Geometry check sheet. Reference: drawing and pictorial views, mm from the part's lowest x, y, z. Round coordinates to 2 decimals unless told otherwise and drop trailing zeros. Write each loop counter-clockwise with the first axis right and the second up, starting at its lowest first coordinate (ties: lowest second). Pieces come first, ordered by that corner, then holes. Notation, with made-up numbers: M 5.25,21 L 56.25,21 A22 ccw 56.25,37 Z; hole C -22,66 d3. An arc over 180 degrees is marked long. One line per item, written item: value. Start each with the question number.
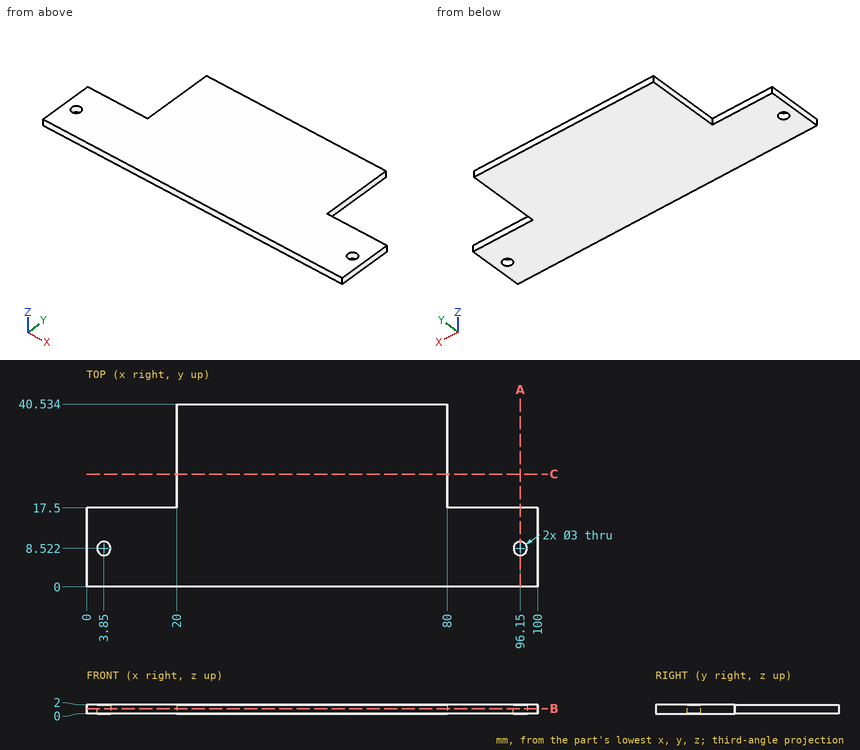
1) Gauge pin test, flat ends, axial feed: pin 1 Ø0.6 at (x, z) = (89, 1) entering from +Y; pin 2 Ø2.5 at (x, y) = (3.85, 8.52) entering from -Z. Record the tip position at first contact, or that the pin passes through.
2) Cross-section at A-A (x = 96.15). Record the boundary of the cut face in (y, z).
3) Cross-section at B-B (z = 1.15). State how many separate pieces and enclosed holes the cut face has, then the cut area to 3 significant figures.
4) Cross-section at C-C (y = 25). Record the boundary of the cut face in (x, z), then the cut area to 3 significant figures.
5) Thickness scan on line 1 (Y direction, x = 96.15, z = 1.4); line 2 (X direction, y = 36, z = 0.5); line 3 (Y direction, x = 90, z = 0.1). Record the ranges inside material, lowest first.
Results below:
1. pin 1: stops at y = 17.5
1. pin 2: passes through
2. outline: M 0,0 L 7.02,0 L 7.02,2 L 0,2 Z; M 10.02,0 L 17.5,0 L 17.5,2 L 10.02,2 Z
3. separate pieces: 1
3. enclosed holes: 2
3. area: 3,120 mm²
4. outline: M 20,0 L 80,0 L 80,2 L 20,2 Z
4. area: 120 mm²
5. line 1: y = 0 to 7.02, 10.02 to 17.5
5. line 2: x = 20 to 80
5. line 3: y = 0 to 17.5
